Build history of the part. All positions in model axes, mm. A direction names the side the tool comes from. Coordinates: 2 decimals unless noted, no trailing zeros. Order: outer loops, then holes, each group sorted by start corner. A loop starts at its lowest first (then second) coordinate and runs counter-clockwise, first axis right, second up. Notation, with made-up numbers: (36.5, 2) - (80.5, 2) arc R10 ccw to (80.5, 16) - close; hole circle Ø9 at (39.25, -17.75). An arc over 180 degrees is marked (long way). Return JSON: item names as keys, results as strings.
Autodesk Inventor part; units mm, degrees
ref_plane "Work Plane1" through (-20.5163, 50.8, -469.9) normal (1, 0, 0) x (0, 0, -1)
ref_plane "YZ Plane" through (0, 0, 0) normal (1, 0, 0) x (0, 1, 0)
ref_plane "XZ Plane" through (0, 0, 0) normal (0, 1, 0) x (-1, 0, 0)
sketch "Sketch1" plane through (0, 0, 0) normal (0, 1, 0) x (-1, 0, 0)
  line L0 (0, 0) -> (0, -469.9)
  line L1 (0, -469.9) -> (0, -122.0086)
  line L2 (0, -469.9) -> (20.5163, -469.9)
  line L3 (20.5163, -469.9) -> (0, 0)
  dimension "d0" = 469.9
  dimension "d1" = 2.5
extrude "Extrusion1" add sketch "Sketch1" along normal blind 50.8
ref_plane "Work Plane1" through (-20.5163, 50.8, -469.9) normal (1, 0, 0) x (0, 0, -1)
sketch "Sketch2" plane through (0, 0, 0) normal (1, 0, 0) x (0, 0, -1)
  line L0 (0, 0) -> (469.9, 0)
  line L1 (0, 50.8) -> (469.9, 50.8)
  line L2 (0, 0) -> (469.9, 0)
  line L3 (469.9, 0) -> (469.9, 50.8)
  line L4 (469.9, 50.8) -> (0, 50.8)
  line L5 (0, 50.8) -> (0, 0)
extrude "Extrusion2" add sketch "Sketch2" along normal blind 12.7
sketch "Sketch4" plane through (-20.5163, 50.8, -469.9) normal (1, 0, 0) x (0, 0, -1)
  line L0 (0, -50.8) -> (0, 0) construction
  line L1 (0, -25.4) -> (-279.4, -25.4) construction
  line L2 (0, -50.8) -> (-469.9, -50.8) construction
  line L3 (-469.9, -50.8) -> (-469.9, 0) construction
  point P0 (-381, -25.4)
  point P1 (-123.825, -25.4)
  point P2 (-469.9, 0)
  dimension "d16" = 25.4
  dimension "d17" = 88.9
  dimension "d18" = 346.075
hole "Hole2" at (-20.5163, 25.4, -88.9) at (-20.5163, 25.4, -346.075) direction (1, 0, 0) diameter 6.7564 end through all
sketch "Sketch6" plane through (-20.5163, 50.8, -469.9) normal (1, 0, 0) x (0, 0, -1)
  circle A0 centre (-123.825, -25.4) radius 3.3782
  line L0 (-130.2408, -25.4) -> (-127.0329, -19.8438)
  line L1 (-127.0329, -19.8438) -> (-120.6171, -19.8438)
  line L2 (-120.6171, -19.8438) -> (-117.4092, -25.4)
  line L3 (-117.4092, -25.4) -> (-120.6171, -30.9563)
  line L4 (-120.6171, -30.9563) -> (-127.0329, -30.9562)
  line L5 (-127.0329, -30.9562) -> (-130.2408, -25.4)
  circle A1 centre (-381, -25.4) radius 3.3782
  line L6 (-387.4158, -25.4) -> (-384.2079, -19.8438)
  line L7 (-384.2079, -19.8438) -> (-377.7921, -19.8438)
  line L8 (-377.7921, -19.8438) -> (-374.5842, -25.4)
  line L9 (-374.5842, -25.4) -> (-377.7921, -30.9563)
  line L10 (-377.7921, -30.9563) -> (-384.2079, -30.9563)
  line L11 (-384.2079, -30.9563) -> (-387.4158, -25.4)
  line L12 (0, 0) -> (-469.9, 0)
  point P0 (-469.9, -50.8)
  dimension "d26" = 11.1125
extrude "Extrusion3" cut sketch "Sketch6" along normal blind 23.368
ref_plane "Work Plane2" through (-20.5163, 0, -234.95) normal (0, 0, -1) x (-1, 0, 0)
sketch "Sketch8" plane through (-20.5163, 50.8, -469.9) normal (1, 0, 0) x (0, 0, -1)
  circle A0 centre (-123.825, -25.4) radius 3.3782 construction
  circle A1 centre (-381, -25.4) radius 3.3782 construction
  line L0 (-123.825, -25.4) -> (-381, -25.4) construction
  line L1 (0, 0) -> (-469.9, 0) construction
  line L2 (-234.95, 0) -> (-234.95, -50.8) construction
  line L3 (-158.75, -38.1) -> (-311.15, -38.1)
  line L4 (-311.15, -38.1) -> (-311.15, -12.7)
  line L5 (-311.15, -12.7) -> (-158.75, -12.7)
  line L6 (-158.75, -12.7) -> (-158.75, -38.1)
  line L7 (-158.75, -38.1) -> (-311.15, -12.7) construction
  line L8 (-311.15, -38.1) -> (-158.75, -12.7) construction
  point P0 (-469.9, -50.8)
  point P1 (-234.95, -25.4)
  dimension "d30" = 25.4
  dimension "d31" = 152.4
extrude "Extrusion4" cut sketch "Sketch8" along normal through all
equation "\"d0\" = lengthOfFixture"
equation "\"d1\" = cutAngle"
equation "\"d2\" = heightOfJig"
equation "\"d4\" = addedDepthToSupportBolts"
equation "\"d16\" = heightOfBoltHolt"
equation "\"d26\" = hexBoltDiameter"
equation "\"d27\" = depthOfHoleForHexBolt + clearanceForHexbolt"
equation "\"lengthOfFixture\" = 469.9"
equation "\"cutAngle\" = 2.5deg"
equation "\"bottomToFirstHole\" = 88.9"
equation "\"distanceBetweenBolts\" = 257.175"
equation "\"bottomToSecondHole\" = bottomToFirstHole + distanceBetweenBolts"
equation "\"heightOfBoltHolt\" = 25.4"
equation "\"boltSize\" = 6.35"
equation "\"heightOfJig\" = 50.8"
equation "\"addedDepthToSupportBolts\" = 12.7"
equation "\"depthOfHoleForHexBolt\" = 22.86"
equation "\"hexBoltDiameter\" = 11.1125"
equation "\"clearanceForHexbolt\" = 0.508"
equation "\"d29\" = -0.5 * lengthOfFixture"
properties part number "jigForRipCuts" material "PC/ABS Plastic"
1. Drop flat-ended pins along their axis: pin 1 (11 mm diameter, centred on y = 25.4, z = -88.9, fed in from -X); pin 2 (12 mm diameter, centred on y = 27, z = -345.5, fed in from -X); pin 3 (6 mm diameter, centred on y = 35, z = -327.5, fed in from -X). Give the stop position or say it passes through.
Check values:
{"pin 1": "x = 2.85", "pin 2": "x = -15.35", "pin 3": "x = -14.43"}
2. Probe L1, parallel to Z at x = 9.25, y = 25.4; L2, parallel to Z at x = 8, y = 25; L3, parallel to Y at x = -6.5, z = -348.5. List the from-to ranges inside material, lowest first.
Check values:
{"L1": "-469.9 to -349.45, -342.7 to -311.15, -158.75 to -92.28, -85.52 to 0", "L2": "-469.9 to -349.43, -342.72 to -311.15, -158.75 to -92.25, -85.55 to 0", "L3": "0 to 19.84, 30.96 to 50.8"}
3. Cut at B-B on z = -301.5. Give the cut face in (x, y), plus the area to 3 significant figures.
Check values:
{"outline": "(-13.16, 0) - (12.7, 0) - (12.7, 12.7) - (-13.16, 12.7) - close; (-13.16, 38.1) - (12.7, 38.1) - (12.7, 50.8) - (-13.16, 50.8) - close", "area": "657 mm²"}
4. Tool access for faces 5 (the flat face through (2.852, 28, -92)), 6 (the flat face through (-10.4, 42, -238.2)), 7 (the flat face through (-1, 26, -311.15)): list every direction of +Z, -Z, +X, -X, +Y, -Y with a clear straight run to the whole face (end or side of a thin tool).
Check values:
{"face 5": "-X", "face 6": "+Z, -X, +Y, -Y", "face 7": "+X, -X"}
5. Cut at A-A on z = -208. Give the cut face in (x, y).
Check values:
{"outline": "(-9.08, 0) - (12.7, 0) - (12.7, 12.7) - (-9.08, 12.7) - close; (-9.08, 38.1) - (12.7, 38.1) - (12.7, 50.8) - (-9.08, 50.8) - close"}
6. Cut at C-C on z = -122.5. Give the cut face in (x, y), plus the area to 3 significant figures.
Check values:
{"outline": "(-5.35, 0) - (12.7, 0) - (12.7, 50.8) - (-5.35, 50.8) - close", "area": "917 mm²"}
7. Mould opens along Z. For faces 1 (the flat face through (0, 0, -284)), 2 (the flat face through (6, 26, 0)), 3 (the flat face through (2, 12.7, -236)), 4 (the flat face through (-4, 25, -469.9)) say: pulls with the +Z half, pulls with the -Z half, needs draft (parallel to the pull), parting line crosses it, or undercut.
Check values:
{"face 1": "needs draft", "face 2": "pulls with the +Z half", "face 3": "undercut", "face 4": "pulls with the -Z half"}
